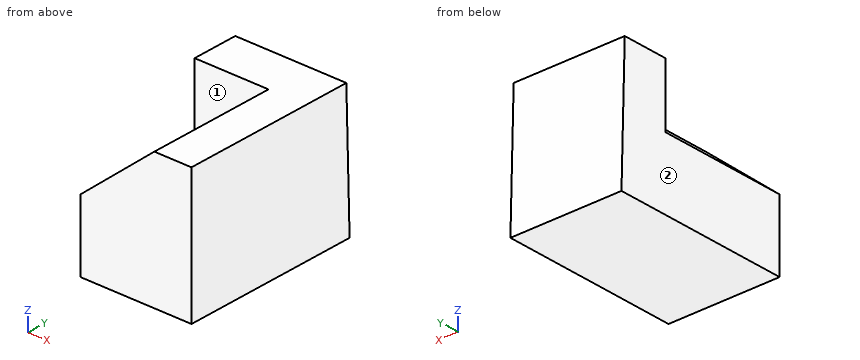
from build123d import *

# Parameters (mm, degrees)
F1_DEPTH = 65.024
F3_DEPTH = 75.946


with BuildPart() as f1:
    # F0 (on Right) → F1 (new body)
    with BuildSketch(Plane.YZ):
        Polygon((46.052266, 37.058897), (-56.906339, 37.058897), (-56.906339, -41.400526), (48.223082, -41.400526), align=None)
    extrude(amount=F1_DEPTH)

    # F2 (on face) → F3 (cut)
    with BuildSketch(Plane.XZ.offset(56.906339)):
        Polygon((0, 0), (43.261223, 37.058897), (0, 37.058897), align=None)
    extrude(amount=-F3_DEPTH, mode=Mode.SUBTRACT)


solid = f1.part
For this review, take the finished solid that the model builds, in its own axes (mm). Face numbers are marked on the shaded views. A direction names the side the tool comes from. Round coordinates to 2 decimals unless told otherwise and drop trailing zeros. Order: outer loops, then holes, each group sorted by start corner. A loop starts at its lowest first (then second) coordinate and runs counter-clockwise, first axis right, second up. Notation, with made-up numbers: (19.5, 19.5) -> (53.5, 19.5) arc R20 cw to (53.5, 54.5) -> close; hole circle Ø5 at (9.5, -35.5). An arc over 180 degrees is marked (long way). Write item = value, one per line. Start each with the question number.
1) Insertion check: pin 1 (3 mm diameter, centred on x = 15, z = 21, fed in from -Y); pin 2 (1 mm diameter, centred on x = 43, y = 5.5, fed in from +Z); pin 3 (1 mm diameter, centred on x = 20.5, z = -0.5, fed in from +Y); pin 4 (1 mm diameter, centred on x = 53, z = -7.5, fed in from +Y). Each pin has a flat end and moves straight along its axis. Give the tip position at first contact, or say it passes through.
2) To check wall thickness, follow line 1 (Y direction, x = 45, z = -23.5); line 2 (Y direction, x = 30.5, z = 33.5); line 3 (Z direction, x = 15, y = -34). State the ranges of each line that lie inside material, in increasing order. Write a range as from..to.
3) Take a section at C-C on z = 17.5. State the section outline as (x, y) points, plus the area to 3 significant figures.
4) Take a section at A-A on y = -35. State the section outline as (x, z) points, plus the area to 3 significant figures.
5) Take a section at B-B on x = 4.5. State the section outline as (y, z) points.
6) Tool access review of the marked faces 1 and 2: name each direction out of +Z, -Z, +X, -X, +Y, -Y from which nothing blocks a thin tool from reaching the whole face with its end or side.
Verdict:
q1.pin_1 = 19.04
q1.pin_2 = 37.06
q1.pin_3 = 47.11
q1.pin_4 = 47.3
q2.line_1 = -56.91..47.73
q2.line_2 = 19.04..46.15
q2.line_3 = -41.4..12.85
q3.outline = (0, 19.04) -> (20.43, 19.04) -> (20.43, -56.91) -> (65.02, -56.91) -> (65.02, 46.59) -> (0, 46.59) -> close
q3.area = 5,180 mm2
q4.outline = (0, -41.4) -> (65.02, -41.4) -> (65.02, 37.06) -> (43.26, 37.06) -> (0, 0) -> close
q4.area = 4,300 mm2
q5.outline = (-56.91, -41.4) -> (48.22, -41.4) -> (46.05, 37.06) -> (19.04, 37.06) -> (19.04, 3.85) -> (-56.91, 3.85) -> close
q6.face_1 = +Z, -X, -Y
q6.face_2 = +Z, -Z, -X, +Y, -Y
